Input: part model. Units: mm. Frame: model coordinates. Face numbers are marked on the shaded views. A direction names the side the tool comes from. Give positions to 0.01 mm unless a question says otherwise; leave off trailing zeros. Write each loop counter-clockwise with the first axis right and the second up, starting at its lowest first coordinate (ties: lowest second). Pieces come first, ordered by that corner, then holes. Notation, with made-up numbers: (65, 60.25) - (112, 60.25) arc R18 ccw to (112, 75.25) - close; hole circle Ø3 at (71, 43.25). An arc over 180 degrees is marked (long way). Answer as a JSON object with one key per item and string values. Group by question number.
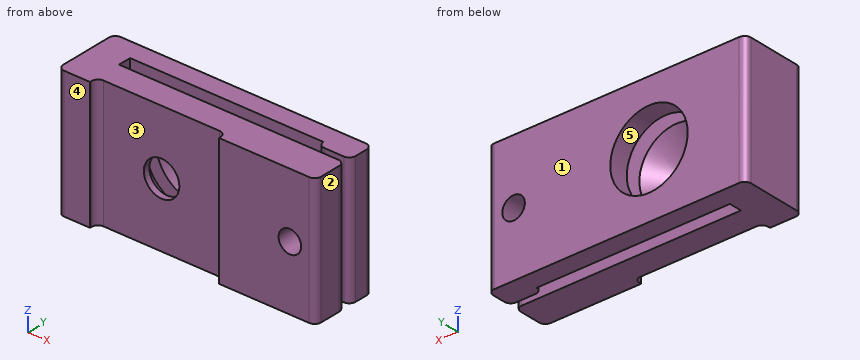
from build123d import *

# Parameters (mm, degrees)
F0_W     = 5
F0_H     = 2
F0_H_2   = 1.2903230384
F0_W_2   = 15
F0_H_3   = 1
F1_DEPTH = 20
F2_R     = 2.75
F2_R_2   = 1.75
F3_DEPTH = 25
F4_R     = 0.99999
F5_R     = 6
F5_R_2   = 2.75
F6_DEPTH = 5
F7_SIZE  = 3


# Not quite as in the source:
# - a fillet or chamfer is up to 0.001 mm smaller than in the source, because OpenCascade refuses the exact size


with BuildPart() as f1:
    # F0 (on Top) → F1 (new body)
    with BuildSketch(Plane.XY):
        Polygon((27.1122940337, 4), (-12.8877059663, 4), (-12.8877059663, 1), (-7.8877059663, 1), (22.1122940337, 1), (27.1122940337, 1), align=None)
        with Locations((-10.3877059663, 0)):
            Rectangle(F0_W, F0_H)
        Polygon((-7.8877059663, -1), (-12.8877059663, -1), (-12.8877059663, -5), (-7.8877059663, -5), (12.1122940337, -5), (27.1122940337, -5), (27.1122940337, -1), align=None)
        with Locations((-10.3877059663, -5.6451615192)):
            Rectangle(F0_W, F0_H_2)
        with Locations((19.6122940337, -5.6451615192)):
            Rectangle(F0_W_2, F0_H_2)
        with Locations((24.6122940337, 0.5)):
            Rectangle(F0_W, F0_H_3)
    extrude(amount=F1_DEPTH)

    # F2 (on face) → F3 (cut)
    with BuildSketch(Plane(origin=(0, 4, 0), x_dir=(-1, 0, 0), z_dir=(0, 1, 0))):
        with Locations((-2.1122940337, 10)):
            Circle(F2_R)
        with Locations((-23.1122940337, 10)):
            Circle(F2_R_2)
    extrude(amount=-F3_DEPTH, mode=Mode.SUBTRACT)

    # F4 (radius 1 in the source; OpenCascade refuses exactly that, so slightly less here)
    f4_edges = [f1.edges().sort_by_distance(p)[0] for p in [
        (-7.887706, -5, 10),
        (12.112294, -5, 10),
        (-12.887706, -6.290323, 10),
        (27.112294, -6.290323, 10),
        (27.112294, -1, 10),
        (27.112294, 0, 10),
        (27.112294, 4, 10),
        (-12.887706, 4, 10),
        (22.112294, 0, 15.71807),
        (22.112294, 0, 4.28193),
    ]]
    fillet(f4_edges, radius=F4_R)

    # F5 (on face) → F6 (cut)
    with BuildSketch(Plane(origin=(0, 4, 0), x_dir=(-1, 0, 0), z_dir=(0, 1, 0))):
        with Locations((-2.1122940337, 10)):
            Circle(F5_R)
        with Locations((-2.1122940337, 10)):
            Circle(F5_R_2, mode=Mode.SUBTRACT)
    extrude(amount=-F6_DEPTH, mode=Mode.SUBTRACT)

    # F7
    f7_edges = [f1.edges().sort_by_distance(p)[0] for p in [
        (4.862294, -1, 10),
    ]]
    chamfer(f7_edges, length=F7_SIZE)


solid = f1.part
1) Pin query (flat end, axial travel): P1, Ø5, axis at x = -1.5, y = -0.5, coming from the +Z side; P2, Ø9, axis at x = 2.11, z = 10, coming from the -Y side. Return the tip coordinate at first contact, or that it passes through.
2) Cut plane C-C on y = -3.5. Return the cut outline in (x, z).
3) Cut plane B-B on z = 10. Count the separate pieces of the cut face and the enclosed holes in it, and give its area (3 significant figures).
4) Reachability of the marked faces 4 and 5 from +Z, -Z, +X, -X, +Y, -Y: full face, straight path, thin tool, end or side. Return the list, or none.
5) Cut plane A-A on x = 19.5. Return the cut outline in (y, z).
6) Line query: line 1 along Y through (x, z) = (16, 17); line 2 along Y through (x, z) = (9.5, 18.75); line 3 along Z through (x, y) = (-2.5, 1.5). Output: solid intervals per line, ascending. Write a range as from..to.
7) Mould query, pull axis X, two halves, no side actions, for the marked faces 1, 2 and 3. Classes: +X half, -X half, draft (parallel to the pull), parting line (faces both ways), or undercut.
Filled in:
{
 "1": {"P1": "stops at z = 20", "P2": "stops at y = -5"},
 "2": {"outline": "(-12.89, 0) - (27.11, 0) - (27.11, 20) - (-12.89, 20) - close; hole circle Ø6.5 at (2.11, 10); hole circle Ø3.5 at (23.11, 10)"},
 "3": {"separate pieces": "5", "enclosed holes": "0", "area": "221 mm²"},
 "4": {"face 4": "+Z, -Z, +X, -X, -Y", "face 5": "+Y"},
 "5": {"outline": "(-6.29, 0) - (-1, 0) - (-1, 20) - (-6.29, 20) - close; (1, 0) - (4, 0) - (4, 20) - (1, 20) - close"},
 "6": {"line 1": "y = -6.29..-1, 1..4", "line 2": "y = -5..-1, 1..4", "line 3": "z = 0..6.16, 13.84..20"},
 "7": {"face 1": "draft", "face 2": "+X half", "face 3": "undercut"}
}
